```python
from build123d import *

# Parameters (mm, degrees)
SKETCH2_R           = 24
SKETCH2_R_2         = 18
BOSS_EXTRUDE2_DEPTH = 9
BOSS_EXTRUDE3_START = 2
SKETCH2_3_R         = 18
SKETCH2_3_R_2       = 16
SKETCH2_3_R_3       = 3.5
SKETCH2_3_R_4       = 4
BOSS_EXTRUDE3_DEPTH = 7
CHAMFER1_SIZE       = 1
CHAMFER2_SIZE       = 2


with BuildPart() as part:
    # Sketch2 → Boss-Extrude2 (new body)
    with BuildSketch(Plane(origin=(0, 0, 0), x_dir=(1, 0, 0), z_dir=(0, 1, 0))):
        with Locations(Location((0, 0, 0), (0, 0, 270))):
            Circle(SKETCH2_R)
        with Locations(Location((0, 0, 0), (0, 0, 270))):
            Circle(SKETCH2_R_2, mode=Mode.SUBTRACT)
    extrude(amount=BOSS_EXTRUDE2_DEPTH)

    # Sketch2<3> → Boss-Extrude3 (add)
    # profile 1 of 2: a face of its own
    with BuildSketch(Plane(origin=(0, 0, 0), x_dir=(1, 0, 0), z_dir=(0, 1, 0)).offset(BOSS_EXTRUDE3_START)):
        with Locations(Location((0, 0, 0), (0, 0, 270))):
            Circle(SKETCH2_3_R)
        Circle(SKETCH2_3_R_2, mode=Mode.SUBTRACT)
    # profile 2 of 2: a face of its own
    with BuildSketch(Plane(origin=(0, 0, 0), x_dir=(1, 0, 0), z_dir=(0, 1, 0)).offset(BOSS_EXTRUDE3_START)):
        Circle(SKETCH2_3_R_2)
        with Locations(Location((-12, 0, 0), (0, 0, 270))):
            Circle(SKETCH2_3_R_3, mode=Mode.SUBTRACT)
        with Locations(Location((0, -12, 0), (0, 0, 270))):
            Circle(SKETCH2_3_R_3, mode=Mode.SUBTRACT)
        with Locations(Location((12, 0, 0), (0, 0, 270))):
            Circle(SKETCH2_3_R_3, mode=Mode.SUBTRACT)
        with Locations(Location((0, 12, 0), (0, 0, 270))):
            Circle(SKETCH2_3_R_3, mode=Mode.SUBTRACT)
        with Locations(Location((0, 0, 0), (0, 0, 270))):
            Circle(SKETCH2_3_R_4, mode=Mode.SUBTRACT)
    extrude(amount=BOSS_EXTRUDE3_DEPTH)

    # Chamfer1
    chamfer1_edges = [part.edges().sort_by_distance(p)[0] for p in [
        (0, 9, -24),
        (0, 0, -24),
    ]]
    chamfer(chamfer1_edges, length=CHAMFER1_SIZE)

    # Chamfer2
    chamfer2_edges = [part.edges().sort_by_distance(p)[0] for p in [
        (0, 2, -18),
    ]]
    chamfer(chamfer2_edges, length=CHAMFER2_SIZE - 0.0001)  # a hair under: the kernel refuses the full size


solid = part.part
```
Work out the finished part from the listing and answer in its coordinate system (mm). A direction names the side the tool comes from. Round coordinates to 2 decimals unless told otherwise and drop trailing zeros. Order: outer loops, then holes, each group sorted by start corner. A loop starts at its lowest first (then second) coordinate and runs counter-clockwise, first axis right, second up.
Q1. A cutting plane is placed at A-A, the plane z = 0. Count the separate pieces of the cut face and the enclosed holes in it, then the cut area to 3 significant figures.
Solution:
separate pieces: 4
enclosed holes: 0
area: 208 mm2
Q2. A cutting plane is placed at C-C, the plane y = 6. Determine the outline of the cut face in (x, z), then the cut area to 3 significant figures.
Solution:
outline: circle Ø48 at (0, 0); hole circle Ø7 at (-12, 0); hole circle Ø8 at (0, 0); hole circle Ø7 at (0, -12); hole circle Ø7 at (0, 12); hole circle Ø7 at (12, 0)
area: 1,610 mm2
Q3. Find the intervals of material crossed by line 1 along Z through (x, y) = (-3, 2.5); line 2 along X through (y, z) = (1.25, 7.5); line 3 along X through (y, z) = (1.5, -4.5), in increasing order.
Solution:
line 1: z = -23.81 to -13.8, -10.2 to -2.65, 2.65 to 10.2, 13.8 to 23.81
line 2: x = -22.8 to -14.98, 14.98 to 22.8
line 3: x = -23.57 to -15.87, 15.87 to 23.57
Q4. The mould has two halves that part along Z. Classify faces 3 (the cylindrical face through (7.21, 4.45, 22.89)), 4 (the cylindrical face through (-15.417, 5.451, -0.759)), 5 (the flat face through (0, 9, 5)): pulls with the +Z half, pulls with the -Z half, needs draft (parallel to the pull), parting line crosses it, or undercut.
Solution:
face 3: parting line crosses it
face 4: undercut
face 5: needs draft
Q5. A tool of negligible diameter and unlimited length cuts with its end or side. For faces 1 (the flat face through (-3, 2, 3)), 2 (the cylindrical face through (0.154, 5.451, 8.503)), from which of +Z, -Z, +X, -X, +Y, -Y can it reach the whole face along a straight path? Write none if from no direction.
Solution:
face 1: -Y
face 2: +Y, -Y
Q6. Given pin 1 Ø4 at (x, z) = (-12, 0) entering from -Y; pin 2 Ø6 at (x, z) = (-6.5, 17) entering from -Y; pin 3 Ø4 at (y, z) = (7.5, 18) entering from -X; pin 4 Ø9.5 at (x, z) = (-2, -3) entering from -Y, each flat-ended and moving along its own axis, determine where each tip first touches the part or whether it passes through.
Solution:
pin 1: passes through
pin 2: stops at y = 0
pin 3: stops at x = -17.89
pin 4: stops at y = 2
